Verification items for the finished model (mm, model axes). A direction names the side the tool comes from. Coordinates: 2 decimals unless noted, no trailing zeros. Write each loop counter-clockwise with the first axis right and the second up, starting at its lowest first coordinate (ties: lowest second). Pieces come first, ordered by that corner, then holes. Notation, with made-up numbers: M 27,72.25 L 83,72.25 A18 cw 83,103.25 Z; hole C -9,86 d1. An arc over 180 degrees is marked long. One line per item, written item: value.
```python
from build123d import *

# Parameters (mm, degrees)
SKETCH_1_W          = 45
SKETCH_1_H          = 16
EXTRUDE_1_DEPTH     = 15
SKETCH_2_W          = 16.428070739
SKETCH_2_H          = 9.700994635
CUT_EXTRUDE_2_DEPTH = 29.200177304
CHAMFER_2_SIZE      = 5
SKETCH_3_R          = 2
CUT_EXTRUDE_3_DEPTH = 30.38537051
SKETCH_4_R          = 2
CUT_EXTRUDE_1_DEPTH = 32.420534687
CHAMFER_13_SIZE     = 3
CHAMFER_14_SIZE     = 15
CHAMFER_14_SIZE2    = 7.975641475
FILLET_5_R          = 6
FILLET_6_R          = 2


with BuildPart() as part:
    # Эскиз1 → Вытянуть1 (new body)
    with BuildSketch(Plane.XY):
        Rectangle(SKETCH_1_W, SKETCH_1_H)
    extrude(amount=EXTRUDE_1_DEPTH)

    # Эскиз2 → Вытянуть2 (cut, through all)
    with BuildSketch(Plane.XY.offset(15)):
        with Locations((-17.390581002, -8.350497318)):
            Rectangle(SKETCH_2_W, SKETCH_2_H)
        with Locations((-17.390581002, 8.350497318)):
            Rectangle(SKETCH_2_W, SKETCH_2_H)
    extrude(amount=-CUT_EXTRUDE_2_DEPTH, mode=Mode.SUBTRACT)

    # Фаска2
    chamfer_2_edges = [part.edges().sort_by_distance(p)[0] for p in [
        (-22.5, 0, 0),
        (-22.5, 0, 15),
    ]]
    chamfer(chamfer_2_edges, length=CHAMFER_2_SIZE)

    # Эскиз3 → Вытянуть3 (cut, through all)
    with BuildSketch(Plane.XZ.offset(3.5)):
        with Locations((-17.875553024, 7.626170468)):
            Circle(SKETCH_3_R)
    extrude(amount=-CUT_EXTRUDE_3_DEPTH, mode=Mode.SUBTRACT)

    # Эскиз4 → Вырез-Вытянуть1 (cut, through all)
    with BuildSketch(Plane(origin=(0, 8, 0), x_dir=(1, 0, 0), z_dir=(0, 1, 0))):
        with Locations(Location((17.10092862, -9.768048927, 0), (0, 0, 270))):
            Circle(SKETCH_4_R)
    extrude(amount=-CUT_EXTRUDE_1_DEPTH, mode=Mode.SUBTRACT)

    # Фаска13
    chamfer_13_edges = [part.edges().sort_by_distance(p)[0] for p in [
        (22.5, 0, 15),
    ]]
    chamfer(chamfer_13_edges, length=CHAMFER_13_SIZE)

    # Фаска14
    chamfer_14_edges = [part.edges().sort_by_distance(p)[0] for p in [
        (22.5, 0, 0),
    ]]
    chamfer_14_side = [part.faces().sort_by_distance(p)[0] for p in [
        (4.599602818, 0, 0),
    ]]
    chamfer(chamfer_14_edges, length=CHAMFER_14_SIZE, length2=CHAMFER_14_SIZE2, reference=chamfer_14_side[0])

    # Скругление5
    # the kernel refuses this fillet: 6 mm, written as the material it adds along each edge
    with BuildSketch(Plane(origin=(-9.176545632, -3.5, 15), x_dir=(0, -1, 0), z_dir=(0, 0, -1))) as fillet_5_piece_1:
        with BuildLine():
            CenterArc((6, 5.809475019), FILLET_5_R, 180, 75.522487814)
            Line((0, 5.809475019), (-0.12, 5.809475019))
            Line((-0.12, 5.809475019), (-0.12, 0))
            Line((-0.12, 0), (0, -0.12))
            ThreePointArc((0, -0.12), (2.25, -0.12), (4.47, -0.1161895))
            Line((4.47, -0.1161895), (4.5, 0))
        make_face()
    extrude(amount=15)
    with BuildSketch(Plane(origin=(-9.176545632, 3.5, 15), x_dir=(0, 1, 0), z_dir=(0, 0, -1))) as fillet_5_piece_2:
        with BuildLine():
            CenterArc((6, -5.809475019), FILLET_5_R, 104.477512186, 75.522487814)
            Line((0, -5.809475019), (-0.12, -5.809475019))
            Line((-0.12, -5.809475019), (-0.12, 0))
            Line((-0.12, 0), (0, 0.12))
            ThreePointArc((0, 0.12), (2.25, 0.12), (4.47, 0.1161895))
            Line((4.47, 0.1161895), (4.5, 0))
        make_face()
    extrude(amount=15)

    # Скругление6
    fillet_6_edges = [part.edges().sort_by_distance(p)[0] for p in [
        (-9.176545632, -8, 7.5),
        (-16.243010326, 3.5, 0),
        (-16.243010326, 3.5, 15),
        (-16.243010326, -3.5, 0),
        (-16.243010326, -3.5, 15),
        (-11.311786037, -4.75658351, 15),
        (-11.311786037, -4.75658351, 0),
        (-11.311786037, 4.75658351, 15),
        (-11.311786037, 4.75658351, 0),
    ]]
    fillet(fillet_6_edges, radius=FILLET_6_R)


solid = part.part
```
Item 1: Go/stop test with flat-tipped pins: P1, Ø6.5, axis at x = -17.88, z = 7.63, coming from the +Y side; P2, Ø8.5, axis at x = -19, z = 10, coming from the -Y side. Record where each tip stops, or that it passes through.
The answers:
P1: stops at y = 3.51
P2: stops at y = -3.5
Item 2: Cross-section at D-D, the plane x = 10. Enter the section's corners in (y, z).
The answers:
outline: M -8,1.33 L 8,1.33 L 8,15 L -8,15 Z
Item 3: Scan lines: line 1 (X direction, y = -1, z = 8.75); line 2 (X direction, y = 6.75, z = 9.5); line 3 (Y direction, x = -20, z = 12). Record each from-to range of solid material in increasing order.
The answers:
line 1: x = -22.5 to -19.53, -16.22 to 15.38, 18.82 to 22.5
line 2: x = -9.65 to 15.12, 19.08 to 22.5
line 3: y = -3.5 to 3.5
Item 4: Draft check along X on faces 4 (the face through (15.1, -0.11, 4.04)), 5 (the face through (-2, 0, 0)), 6 (the face through (-19.874, -0.049, 7.714)). Enter one of: released by +X, released by -X, zero draft, split by the parting line, or undercut.
The answers:
face 4: released by +X
face 5: zero draft
face 6: undercut
Item 5: Cross-section at C-C, the plane z = 11. Enter the section's corners in (x, y) (3 decimals), and give its area (3 significant figures).
The answers:
outline: M -21.5,-3.5 L -14.986,-3.5 A6 cw -9.591,-6.875 A2 ccw -7.792,-8 L 15.525,-8 L 15.525,8 L -9.177,8 A6 cw -14.986,3.5 L -21.5,3.5 Z; M 18.676,-8 L 22.5,-8 L 22.5,8 L 18.676,8 Z
area: 556 mm²
Item 6: Cross-section at B-B, the plane y = 0.75. Enter the section's corners in (x, z), and give its area (3 significant figures).
The answers:
outline: M -22.5,5 L -17.5,0 L 7.5,0 L 22.5,7.98 L 22.5,12 L 19.5,15 L -17.5,15 L -22.5,10 Z; hole C -17.88,7.63 d4; hole C 17.1,9.77 d4
area: 561 mm²
Item 7: Access from +Z, -Z, +X, -X, +Y, -Y to the whole of each face (thin tool, end or side, straight path). Record for faces 1 (the face through (-16.71, 3.15, 0.87)), 2 (the face through (-16.7, -3.1, 14.2)), 3 (the face through (-20, -3.5, 6)).
The answers:
face 1: -Z, -X, +Y
face 2: +Z, -X, -Y
face 3: +Z, -Z, -X, -Y
Item 8: Cross-section at A-A, the plane z = 6.5. Enter the section's corners in (x, y) (3 decimals), and give its area (3 significant figures).
The answers:
outline: M -22.5,-3.5 L -19.528,-3.5 L -19.528,3.5 L -22.5,3.5 Z; M -16.223,-3.5 L -14.986,-3.5 A6 cw -9.591,-6.875 A2 ccw -7.792,-8 L 19.725,-8 L 19.725,8 L -9.177,8 A6 cw -14.986,3.5 L -16.223,3.5 Z
area: 546 mm²
